For this review, take the finished solid that the model builds, in its own axes (mm). Face numbers are marked on the shaded views. A direction names the side the tool comes from. Give positions to 0.01 mm unless a question says otherwise; leave off trailing zeros. Write each loop counter-clockwise with the first axis right and the second up, starting at its lowest first coordinate (ties: lowest second). Pieces come first, ordered by that corner, then holes. Notation, with made-up numbers: M -6,15 L 16,15 A10 cw 16,19 Z; hole C 50.25,-28 d7. An arc over 180 degrees is marked long. One line per item, written item: value. Start each with the question number.
Item 1: Tool access review of the marked faces 1 and 2: name each direction out of +Z, -Z, +X, -X, +Y, -Y from which nothing blocks a thin tool from reaching the whole face with its end or side.
Item 2: Consider section A-A, the plane z = -11. Write out the cut boundary in (x, y), and give its area (3 significant figures).
Item 3: Consider section D-D, the plane y = 5.5. Write out the cut boundary in (x, z).
Item 4: Consider section C-C, the plane z = -45.5. Write out the cut boundary in (x, y).
Item 5: To check wall thickness, follow probe 1 along X at (y, z) = (0.5, 57.48); probe 2 along Z at (x, y) = (78.45, 1.2) (3 decimals); probe 3 along Z at (x, y) = (7.5, 4). State the ranges of each line that lie inside material, in increasing order.
Item 6: Clearance check with flat-ended pins moving along their axes: pin 1 Ø1.2 at (x, z) = (-46.5, -26) entering from -Y; pin 2 Ø0.5 at (x, y) = (11, 1) entering from +Z; pin 3 Ø1 at (x, y) = (-8.5, 4) entering from -Z. State where each tip first meets the part, or that it passes through.
Item 7: Consider section B-B, the plane x = -15.5. Write out the cut boundary in (y, z).
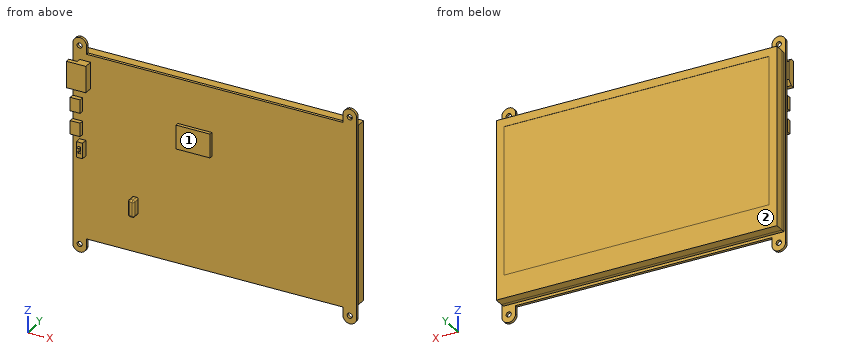
```python
from build123d import *

# Parameters (mm, degrees)
SKETCH_1_W          = 164.9
SKETCH_1_H          = 124.27
EXTRUDE_2_DEPTH     = 1.6
SKETCH_2_W          = 148.9
SKETCH_2_H          = 8.655
CUT_EXTRUDE_1_DEPTH = 104.253671726
SKETCH_3_W          = 163
SKETCH_3_H          = 104
EXTRUDE_4_DEPTH     = 7.5
SKETCH_4_W          = 11.3
SKETCH_4_H          = 15.3
EXTRUDE_5_DEPTH     = 5
SKETCH_6_W          = 3.5
SKETCH_6_H          = 9.85
EXTRUDE_6_DEPTH     = 4.5
FILLET_1_R          = 1
FILLET_2_R          = 1
SKETCH_7_R          = 1.5
CUT_EXTRUDE_3_DEPTH = 105.438837245
FILLET_3_R          = 4
SKETCH_9_W          = 154
SKETCH_9_H          = 86
CUT_EXTRUDE_5_DEPTH = 0.1
CUT_EXTRUDE_6_DEPTH = 5
SKETCH_11_W         = 5.8
SKETCH_11_H         = 7.8
EXTRUDE_7_DEPTH     = 2.6
SKETCH_12_W         = 3.6
SKETCH_12_H         = 9
EXTRUDE_8_DEPTH     = 3.5
SKETCH_13_W         = 1.5
SKETCH_13_H         = 4
CUT_EXTRUDE_7_DEPTH = 0.1
SKETCH_14_W         = 1.5
SKETCH_14_H         = 2
EXTRUDE_9_DEPTH     = 2
SKETCH_15_W         = 19.8
SKETCH_15_H         = 13.8
EXTRUDE_10_DEPTH    = 2
SKETCH_16_W         = 163
SKETCH_16_H         = 104
SKETCH_16_W_2       = 162.8
SKETCH_16_H_2       = 103.8
CUT_EXTRUDE_9_DEPTH = 2.2


# Some blends are built 0.0001 mm under size
with BuildPart() as part:
    # 草图1 → 凸台-拉伸2 (new body)
    with BuildSketch(Plane(origin=(0, 0, 0), x_dir=(1, 0, 0), z_dir=(0, 1, 0))):
        Rectangle(SKETCH_1_W, SKETCH_1_H)
    extrude(amount=EXTRUDE_2_DEPTH)

    # 草图2 → 切除-拉伸1 (cut, through all)
    with BuildSketch(Plane(origin=(0, 1.6, 0), x_dir=(1, 0, 0), z_dir=(0, 1, 0))):
        with Locations((0, 57.8075)):
            Rectangle(SKETCH_2_W, SKETCH_2_H)
        with Locations((0, -57.8075)):
            Rectangle(SKETCH_2_W, SKETCH_2_H)
    extrude(amount=-CUT_EXTRUDE_1_DEPTH, mode=Mode.SUBTRACT)

    # 草图3 → 凸台-拉伸4 (add)
    with BuildSketch(Plane(origin=(0, 1.6, 0), x_dir=(1, 0, 0), z_dir=(0, 1, 0))):
        Rectangle(SKETCH_3_W, SKETCH_3_H)
    extrude(amount=EXTRUDE_4_DEPTH)

    # 草图4 → 凸台-拉伸5 (add)
    with BuildSketch(Plane.XZ):
        with Locations((-77.8, 41.83)):
            Rectangle(SKETCH_4_W, SKETCH_4_H)
    extrude(amount=EXTRUDE_5_DEPTH)

    # 草图6 → 凸台-拉伸6 (add)
    with BuildSketch(Plane(origin=(0, 0, 0), x_dir=(-1, 0, 0), z_dir=(0, -1, 0))):
        with Locations((46.2, 26.555)):
            Rectangle(SKETCH_6_W, SKETCH_6_H)
    extrude(amount=EXTRUDE_6_DEPTH)

    # 圆角1
    fillet_1_edges = [part.edges().sort_by_distance(p)[0] for p in [
        (-44.45, -4.5, -26.555),
        (-46.2, -4.5, -21.63),
        (-47.95, -4.5, -26.555),
        (-46.2, -4.5, -31.48),
    ]]
    fillet(fillet_1_edges, radius=FILLET_1_R)

    # 圆角2
    # the kernel refuses this fillet: 1 mm, written as the material it takes off along each edge
    with BuildSketch(Plane(origin=(-46.95, -3.5, -22.63), x_dir=(0, 0, 1), z_dir=(-1, 0, 0))) as fillet_2_piece_1_section:
        Polygon((0, 0), (FILLET_2_R, 0), (FILLET_2_R, -FILLET_2_R), (0, -FILLET_2_R), align=None)
    fillet_2_piece_1 = extrude(amount=FILLET_2_R, mode=Mode.PRIVATE)
    fillet_2_piece_1 = fillet_2_piece_1 - Plane(origin=(-46.95, -3.5, -22.63), x_dir=(0, 0.7071067811865475, -0.7071067811865475), z_dir=(-1, 0, 0)) * Sphere(FILLET_2_R, mode=Mode.PRIVATE)
    add(fillet_2_piece_1, mode=Mode.SUBTRACT)
    with BuildSketch(Plane(origin=(-45.45, -3.5, -22.63), x_dir=(1, 0, 0), z_dir=(0, 0, 1))) as fillet_2_piece_2_section:
        Polygon((0, 0), (FILLET_2_R, 0), (FILLET_2_R, -FILLET_2_R), (0, -FILLET_2_R), align=None)
    fillet_2_piece_2 = extrude(amount=FILLET_2_R, mode=Mode.PRIVATE)
    fillet_2_piece_2 = fillet_2_piece_2 - Plane(origin=(-45.45, -3.5, -22.63), x_dir=(-0.7071067811865475, 0.7071067811865475, 0), z_dir=(0, 0, 1)) * Sphere(FILLET_2_R, mode=Mode.PRIVATE)
    add(fillet_2_piece_2, mode=Mode.SUBTRACT)
    with BuildSketch(Plane(origin=(-46.95, -3.5, -30.48), x_dir=(0, 0, -1), z_dir=(-1, 0, 0))) as fillet_2_piece_3_section:
        Polygon((0, 0), (FILLET_2_R, 0), (FILLET_2_R, FILLET_2_R), (0, FILLET_2_R), align=None)
    fillet_2_piece_3 = extrude(amount=FILLET_2_R, mode=Mode.PRIVATE)
    fillet_2_piece_3 = fillet_2_piece_3 - Plane(origin=(-46.95, -3.5, -30.48), x_dir=(0, 0.7071067811865475, 0.7071067811865475), z_dir=(-1, 0, 0)) * Sphere(FILLET_2_R, mode=Mode.PRIVATE)
    add(fillet_2_piece_3, mode=Mode.SUBTRACT)
    with BuildSketch(Plane(origin=(-45.45, -3.5, -30.48), x_dir=(1, 0, 0), z_dir=(0, 0, -1))) as fillet_2_piece_4_section:
        Polygon((0, 0), (FILLET_2_R, 0), (FILLET_2_R, FILLET_2_R), (0, FILLET_2_R), align=None)
    fillet_2_piece_4 = extrude(amount=FILLET_2_R, mode=Mode.PRIVATE)
    fillet_2_piece_4 = fillet_2_piece_4 - Plane(origin=(-45.45, -3.5, -30.48), x_dir=(-0.7071067811865475, 0.7071067811865475, 0), z_dir=(0, 0, -1)) * Sphere(FILLET_2_R, mode=Mode.PRIVATE)
    add(fillet_2_piece_4, mode=Mode.SUBTRACT)
    with BuildSketch(Plane(origin=(-44.45, 0, -31.48), x_dir=(-1, 0, 0), z_dir=(0, -1, 0)), Plane(origin=(-47.95, 0, -31.48), x_dir=(0, 0, 1), z_dir=(0, -1, 0))) as fillet_2_piece_5:
        with BuildLine():
            CenterArc((FILLET_2_R, -FILLET_2_R), FILLET_2_R, 90, 90)
            Line((0, -FILLET_2_R), (0, 0))
            Line((0, 0), (FILLET_2_R, 0))
        make_face()
    extrude(amount=3.5, mode=Mode.SUBTRACT)
    with BuildSketch(Plane(origin=(-47.95, 0, -21.63), x_dir=(0, 0, -1), z_dir=(0, -1, 0)), Plane(origin=(-44.45, 0, -21.63), x_dir=(-1, 0, 0), z_dir=(0, -1, 0))) as fillet_2_piece_6:
        with BuildLine():
            CenterArc((FILLET_2_R, FILLET_2_R), FILLET_2_R, 180, 90)
            Line((0, FILLET_2_R), (0, 0))
            Line((0, 0), (FILLET_2_R, 0))
        make_face()
    extrude(amount=3.5, mode=Mode.SUBTRACT)

    # 草图7 → 切除-拉伸3 (cut, through all)
    with BuildSketch(Plane.XZ):
        with Locations(Location((-78.45, 57.48, 0), (0, 0, 270))):
            Circle(SKETCH_7_R)
        with Locations(Location((78.45, 57.48, 0), (0, 0, 90))):
            Circle(SKETCH_7_R)
        with Locations(Location((78.45, -57.48, 0), (0, 0, 270))):
            Circle(SKETCH_7_R)
        with Locations(Location((-78.45, -57.48, 0), (0, 0, 90))):
            Circle(SKETCH_7_R)
    extrude(amount=-CUT_EXTRUDE_3_DEPTH, mode=Mode.SUBTRACT)

    # 圆角3
    fillet_3_edges = [part.edges().sort_by_distance(p)[0] for p in [
        (-74.45, 0.8, -62.135),
        (-82.45, 0.8, -62.135),
        (82.45, 0.8, -62.135),
        (74.45, 0.8, -62.135),
        (74.45, 0.8, 62.135),
        (82.45, 0.8, 62.135),
        (-74.45, 0.8, 62.135),
        (-82.45, 0.8, 62.135),
    ]]
    fillet(fillet_3_edges, radius=FILLET_3_R - 0.0001)  # a hair under: the kernel refuses the full size

    # 草图9 → 切除-拉伸5 (cut)
    with BuildSketch(Plane(origin=(0, 9.1, 0), x_dir=(1, 0, 0), z_dir=(0, 1, 0))):
        with Locations((0, -4.32)):
            Rectangle(SKETCH_9_W, SKETCH_9_H)
    extrude(amount=-CUT_EXTRUDE_5_DEPTH, mode=Mode.SUBTRACT)

    # 草图10 → 切除-拉伸6 (cut)
    with BuildSketch(Plane.ZY.offset(83.45)):
        Polygon((49.48, -2.5), (46.98, 0), (49.48, 0), align=None)
        Polygon((34.18, 0), (34.18, -2.5), (36.68, 0), align=None)
    extrude(amount=-CUT_EXTRUDE_6_DEPTH, mode=Mode.SUBTRACT)

    # 草图11 → 凸台-拉伸7 (add)
    with BuildSketch(Plane.XZ):
        with Locations((-79.65, 23.78)):
            Rectangle(SKETCH_11_W, SKETCH_11_H)
        with Locations((-79.65, 10.28)):
            Rectangle(SKETCH_11_W, SKETCH_11_H)
    extrude(amount=EXTRUDE_7_DEPTH)

    # 草图12 → 凸台-拉伸8 (add)
    with BuildSketch(Plane.XZ):
        with Locations((-76.65, -0.97)):
            Rectangle(SKETCH_12_W, SKETCH_12_H)
    extrude(amount=EXTRUDE_8_DEPTH)

    # 草图13 → 切除-拉伸7 (cut)
    with BuildSketch(Plane.XZ.offset(3.5)):
        with Locations((-76.65, -0.97)):
            Rectangle(SKETCH_13_W, SKETCH_13_H)
    extrude(amount=-CUT_EXTRUDE_7_DEPTH, mode=Mode.SUBTRACT)

    # 草图14 → 凸台-拉伸9 (add)
    with BuildSketch(Plane.XZ.offset(3.4)):
        with Locations((-76.65, 0.03)):
            Rectangle(SKETCH_14_W, SKETCH_14_H)
    extrude(amount=EXTRUDE_9_DEPTH)

    # 草图15 → 凸台-拉伸10 (add)
    with BuildSketch(Plane.XZ):
        with Locations((-11.55, 20.58)):
            Rectangle(SKETCH_15_W, SKETCH_15_H)
    extrude(amount=EXTRUDE_10_DEPTH)

    # 草图16 → 切除-拉伸9 (cut)
    with BuildSketch(Plane(origin=(0, 1.6, 0), x_dir=(1, 0, 0), z_dir=(0, 1, 0))):
        Rectangle(SKETCH_16_W, SKETCH_16_H)
        Rectangle(SKETCH_16_W_2, SKETCH_16_H_2, mode=Mode.SUBTRACT)
    extrude(amount=CUT_EXTRUDE_9_DEPTH, mode=Mode.SUBTRACT)


solid = part.part
```
Model answer:
1. face 1: +Z, -Z, +X, -Y
1. face 2: +Z, -Z, +X, -X, +Y
2. outline: M -82.45,0 L 82.45,0 L 82.45,1.6 L 81.4,1.6 L 81.4,3.8 L 81.5,3.8 L 81.5,9.1 L 77,9.1 L 77,9 L -77,9 L -77,9.1 L -81.5,9.1 L -81.5,3.8 L -81.4,3.8 L -81.4,1.6 L -82.45,1.6 Z
2. area: 1,470 mm2
3. outline: M -81.5,-52 L 81.5,-52 L 81.5,52 L -81.5,52 Z
4. outline: M -82.45,0 L 82.45,0 L 82.45,1.6 L 81.4,1.6 L 81.4,3.8 L 81.5,3.8 L 81.5,9.1 L -81.5,9.1 L -81.5,3.8 L -81.4,3.8 L -81.4,1.6 L -82.45,1.6 Z
5. probe 1: x = -82.45 to -79.95, -76.95 to -74.45, 74.45 to 76.95, 79.95 to 82.45
5. probe 2: z = -62.135 to -58.98, -55.98 to 55.98, 58.98 to 62.135
5. probe 3: z = -52 to 52
6. pin 1: stops at y = -4.5
6. pin 2: stops at z = 53.48
6. pin 3: stops at z = -52
7. outline: M -2,13.68 L 0,13.68 L 0,-53.48 L 1.6,-53.48 L 1.6,-51.9 L 3.8,-51.9 L 3.8,-52 L 9.1,-52 L 9.1,-38.68 L 9,-38.68 L 9,47.32 L 9.1,47.32 L 9.1,52 L 3.8,52 L 3.8,51.9 L 1.6,51.9 L 1.6,53.48 L 0,53.48 L 0,27.48 L -2,27.48 Z
